Build history of the part. All positions in model axes, mm. Coordinates: 2 decimals unless noted, no trailing zeros. Loops run counter-clockwise (first coordinate to the right, second up) from the corner with the lowest first, then second, coordinate; pieces in that order, holes last.
Item 1: Cut at B-B (y = 0.5). Count the separate pieces of the cut face and the enclosed holes in it, and give its area (3 significant figures).
Item 2: Drill centre lines: line 1 along X through (y, z) = (0.7, -80.5); line 2 along Z through (x, y) = (-36.5, 2.55); line 3 along Z through (x, y) = (-81, 2.4). Where is each one in solid material? Low to high.
Item 3: Cut at A-A (z = -94.5). List the corners of the cut face in (x, y), and give its area (3 significant figures).
Item 4: Mould opens along Z. For faces 1 (the face through (-70.09, 1.48, 41.65)), 2 (the face through (2, 0, 24)), 3 (the face through (-17.75, 1.479, -38.065)) say: released by +Z, released by -Z, zero draft, split by the parting line, or undercut.
Item 5: Flat gauge pin, fed straight in: pin 1 (1.5 mm diameter, centred on x = 5, y = 2.5, fed in from +Z). Where does the tip first touch, or does it go through?
from build123d import *

# Parameters (mm, degrees)
SKETCH1_R           = 115
SKETCH1_R_2         = 1.5
SKETCH1_R_3         = 2
SKETCH1_R_4         = 15
BOSS_EXTRUDE3_DEPTH = 3


with BuildPart() as part:
    # Sketch1 → Boss-Extrude3 (new body)
    with BuildSketch(Plane(origin=(0, 0, 0), x_dir=(1, 0, 0), z_dir=(0, 1, 0))):
        with Locations(Location((0, 0, 0), (0, 0, 270))):
            Circle(SKETCH1_R)
        with Locations(Location((-65, 65, 0), (0, 0, 270))):
            Circle(SKETCH1_R_2, mode=Mode.SUBTRACT)
        with Locations(Location((-47.039487758, 27.039487758, 0), (0, 0, 270))):
            Circle(SKETCH1_R_2, mode=Mode.SUBTRACT)
        with Locations(Location((65, 65, 0), (0, 0, 270))):
            Circle(SKETCH1_R_2, mode=Mode.SUBTRACT)
        with Locations(Location((27.039487758, 47.039487758, 0), (0, 0, 270))):
            Circle(SKETCH1_R_2, mode=Mode.SUBTRACT)
        with Locations(Location((15.25, 15.25, 0), (0, 0, 270))):
            Circle(SKETCH1_R_2, mode=Mode.SUBTRACT)
        with Locations(Location((22, 22, 0), (0, 0, 270))):
            Circle(SKETCH1_R_3, mode=Mode.SUBTRACT)
        with Locations(Location((37.039487758, 55.539487758, 0), (0, 0, 270))):
            Circle(SKETCH1_R_2, mode=Mode.SUBTRACT)
        with Locations(Location((37.039487758, 38.539487758, 0), (0, 0, 270))):
            Circle(SKETCH1_R_2, mode=Mode.SUBTRACT)
        with Locations(Location((65, -65, 0), (0, 0, 270))):
            Circle(SKETCH1_R_2, mode=Mode.SUBTRACT)
        with Locations(Location((47.039487758, -27.039487758, 0), (0, 0, 270))):
            Circle(SKETCH1_R_2, mode=Mode.SUBTRACT)
        with Locations(Location((15.25, -15.25, 0), (0, 0, 270))):
            Circle(SKETCH1_R_2, mode=Mode.SUBTRACT)
        with Locations(Location((22, -22, 0), (0, 0, 270))):
            Circle(SKETCH1_R_3, mode=Mode.SUBTRACT)
        with Locations(Location((55.539487758, -37.039487758, 0), (0, 0, 270))):
            Circle(SKETCH1_R_2, mode=Mode.SUBTRACT)
        with Locations(Location((38.539487758, -37.039487758, 0), (0, 0, 270))):
            Circle(SKETCH1_R_2, mode=Mode.SUBTRACT)
        with Locations(Location((-65, -65, 0), (0, 0, 270))):
            Circle(SKETCH1_R_2, mode=Mode.SUBTRACT)
        with Locations(Location((0, 0, 0), (0, 0, 270))):
            Circle(SKETCH1_R_4, mode=Mode.SUBTRACT)
        with Locations(Location((-15.25, 15.25, 0), (0, 0, 270))):
            Circle(SKETCH1_R_2, mode=Mode.SUBTRACT)
        with Locations(Location((-22, 22, 0), (0, 0, 270))):
            Circle(SKETCH1_R_3, mode=Mode.SUBTRACT)
        with Locations(Location((-55.539487758, 37.039487758, 0), (0, 0, 270))):
            Circle(SKETCH1_R_2, mode=Mode.SUBTRACT)
        with Locations(Location((-27.039487758, -47.039487758, 0), (0, 0, 270))):
            Circle(SKETCH1_R_2, mode=Mode.SUBTRACT)
        with Locations(Location((-15.25, -15.25, 0), (0, 0, 270))):
            Circle(SKETCH1_R_2, mode=Mode.SUBTRACT)
        with Locations(Location((-22, -22, 0), (0, 0, 270))):
            Circle(SKETCH1_R_3, mode=Mode.SUBTRACT)
        with Locations(Location((-37.039487758, -55.539487758, 0), (0, 0, 270))):
            Circle(SKETCH1_R_2, mode=Mode.SUBTRACT)
        with Locations(Location((-37.039487758, -38.539487758, 0), (0, 0, 270))):
            Circle(SKETCH1_R_2, mode=Mode.SUBTRACT)
        with Locations(Location((29, 24.5, 0), (0, 0, 90))):
            Circle(SKETCH1_R_2, mode=Mode.SUBTRACT)
        with Locations(Location((29, -24.5, 0), (0, 0, 270))):
            Circle(SKETCH1_R_2, mode=Mode.SUBTRACT)
        with Locations(Location((-29, -24.5, 0), (0, 0, 90))):
            Circle(SKETCH1_R_2, mode=Mode.SUBTRACT)
        with Locations(Location((-29, 24.5, 0), (0, 0, 270))):
            Circle(SKETCH1_R_2, mode=Mode.SUBTRACT)
        with Locations(Location((-38.539487758, 37.039487758, 0), (0, 0, 270))):
            Circle(SKETCH1_R_2, mode=Mode.SUBTRACT)
        with BuildLine():
            Line((26.808945881, 12.501216771), (49.6405219, 23.147755517))
            ThreePointArc((49.6405219, 23.147755517), (53.675730643, 23.232000867), (56.458487137, 20.308599907))
            ThreePointArc((56.458487137, 20.308599907), (60, 0), (56.458487137, -20.308599907))
            ThreePointArc((56.458487137, -20.308599907), (53.675730643, -23.232000867), (49.6405219, -23.147755517))
            Line((49.6405219, -23.147755517), (26.808945881, -12.501216771))
            ThreePointArc((26.808945881, -12.501216771), (24.383041239, -10.066703292), (24.101697658, -6.641398197))
            ThreePointArc((24.101697658, -6.641398197), (25, 0), (24.101697658, 6.641398197))
            ThreePointArc((24.101697658, 6.641398197), (24.383041239, 10.066703292), (26.808945881, 12.501216771))
        make_face(mode=Mode.SUBTRACT)
        with BuildLine():
            Line((67.821864521, 31.625854817), (90.517419336, 42.208965833))
            ThreePointArc((90.517419336, 42.208965833), (94.457574862, 42.331654691), (97.262036177, 39.561298243))
            ThreePointArc((97.262036177, 39.561298243), (104.05397345, -14.063093872), (83.270844776, -63.960662992))
            ThreePointArc((83.270844776, -63.960662992), (78.486399596, -65.847357267), (74.568650349, -62.515425125))
            Line((74.568650349, -62.515425125), (64.070056019, -31.443439938))
            ThreePointArc((64.070056019, -31.443439938), (63.811318327, -29.63450173), (64.219840648, -27.853403152))
            ThreePointArc((64.219840648, -27.853403152), (69.986267395, -1.386497808), (65.272625441, 25.288028156))
            ThreePointArc((65.272625441, 25.288028156), (65.296141705, 28.960167834), (67.821864521, 31.625854817))
        make_face(mode=Mode.SUBTRACT)
        with BuildLine():
            Line((12.501216771, -26.808945881), (23.147755517, -49.6405219))
            ThreePointArc((23.147755517, -49.6405219), (23.232000867, -53.675730643), (20.308599907, -56.458487137))
            ThreePointArc((20.308599907, -56.458487137), (0, -60), (-20.308599907, -56.458487137))
            ThreePointArc((-20.308599907, -56.458487137), (-23.232000867, -53.675730643), (-23.147755517, -49.6405219))
            Line((-23.147755517, -49.6405219), (-12.501216771, -26.808945881))
            ThreePointArc((-12.501216771, -26.808945881), (-10.066703292, -24.383041239), (-6.641398197, -24.101697658))
            ThreePointArc((-6.641398197, -24.101697658), (0, -25), (6.641398197, -24.101697658))
            ThreePointArc((6.641398197, -24.101697658), (10.066703292, -24.383041239), (12.501216771, -26.808945881))
        make_face(mode=Mode.SUBTRACT)
        with BuildLine():
            Line((-26.808945881, -12.501216771), (-49.6405219, -23.147755517))
            ThreePointArc((-49.6405219, -23.147755517), (-53.675730643, -23.232000867), (-56.458487137, -20.308599907))
            ThreePointArc((-56.458487137, -20.308599907), (-60, 0), (-56.458487137, 20.308599907))
            ThreePointArc((-56.458487137, 20.308599907), (-53.675730643, 23.232000867), (-49.6405219, 23.147755517))
            Line((-49.6405219, 23.147755517), (-26.808945881, 12.501216771))
            ThreePointArc((-26.808945881, 12.501216771), (-24.383041239, 10.066703292), (-24.101697658, 6.641398197))
            ThreePointArc((-24.101697658, 6.641398197), (-25, 0), (-24.101697658, -6.641398197))
            ThreePointArc((-24.101697658, -6.641398197), (-24.383041239, -10.066703292), (-26.808945881, -12.501216771))
        make_face(mode=Mode.SUBTRACT)
        with BuildLine():
            Line((-12.501216771, 26.808945881), (-23.147755517, 49.6405219))
            ThreePointArc((-23.147755517, 49.6405219), (-23.232000867, 53.675730643), (-20.308599907, 56.458487137))
            ThreePointArc((-20.308599907, 56.458487137), (0, 60), (20.308599907, 56.458487137))
            ThreePointArc((20.308599907, 56.458487137), (23.232000867, 53.675730643), (23.147755517, 49.6405219))
            Line((23.147755517, 49.6405219), (12.501216771, 26.808945881))
            ThreePointArc((12.501216771, 26.808945881), (10.066703292, 24.383041239), (6.641398197, 24.101697658))
            ThreePointArc((6.641398197, 24.101697658), (0, 25), (-6.641398197, 24.101697658))
            ThreePointArc((-6.641398197, 24.101697658), (-10.066703292, 24.383041239), (-12.501216771, 26.808945881))
        make_face(mode=Mode.SUBTRACT)
        with BuildLine():
            Line((31.625854817, -67.821864521), (42.208965833, -90.517419336))
            ThreePointArc((42.208965833, -90.517419336), (42.331654691, -94.457574862), (39.561298243, -97.262036177))
            ThreePointArc((39.561298243, -97.262036177), (-14.063093872, -104.05397345), (-63.960662992, -83.270844776))
            ThreePointArc((-63.960662992, -83.270844776), (-65.847357267, -78.486399596), (-62.515425125, -74.568650349))
            Line((-62.515425125, -74.568650349), (-31.443439938, -64.070056019))
            ThreePointArc((-31.443439938, -64.070056019), (-29.63450173, -63.811318327), (-27.853403152, -64.219840648))
            ThreePointArc((-27.853403152, -64.219840648), (-1.386497808, -69.986267395), (25.288028156, -65.272625441))
            ThreePointArc((25.288028156, -65.272625441), (28.960167834, -65.296141705), (31.625854817, -67.821864521))
        make_face(mode=Mode.SUBTRACT)
        with BuildLine():
            Line((-67.821864521, -31.625854817), (-90.517419336, -42.208965833))
            ThreePointArc((-90.517419336, -42.208965833), (-94.457574862, -42.331654691), (-97.262036177, -39.561298243))
            ThreePointArc((-97.262036177, -39.561298243), (-104.05397345, 14.063093872), (-83.270844776, 63.960662991))
            ThreePointArc((-83.270844776, 63.960662991), (-78.486399596, 65.847357267), (-74.568650349, 62.515425125))
            Line((-74.568650349, 62.515425125), (-64.070056019, 31.443439938))
            ThreePointArc((-64.070056019, 31.443439938), (-63.811318327, 29.63450173), (-64.219840648, 27.853403152))
            ThreePointArc((-64.219840648, 27.853403152), (-69.986267395, 1.386497808), (-65.272625441, -25.288028156))
            ThreePointArc((-65.272625441, -25.288028156), (-65.296141705, -28.960167834), (-67.821864521, -31.625854817))
        make_face(mode=Mode.SUBTRACT)
        with BuildLine():
            Line((-31.625854817, 67.821864521), (-42.208965833, 90.517419336))
            ThreePointArc((-42.208965833, 90.517419336), (-42.331654691, 94.457574862), (-39.561298243, 97.262036177))
            ThreePointArc((-39.561298243, 97.262036177), (14.063093872, 104.05397345), (63.960662992, 83.270844776))
            ThreePointArc((63.960662992, 83.270844776), (65.847357267, 78.486399596), (62.515425125, 74.568650349))
            Line((62.515425125, 74.568650349), (31.443439938, 64.070056019))
            ThreePointArc((31.443439938, 64.070056019), (29.63450173, 63.811318327), (27.853403152, 64.219840648))
            ThreePointArc((27.853403152, 64.219840648), (1.386497808, 69.986267395), (-25.288028156, 65.272625441))
            ThreePointArc((-25.288028156, 65.272625441), (-28.960167834, 65.296141705), (-31.625854817, 67.821864521))
        make_face(mode=Mode.SUBTRACT)
        with BuildLine():
            ThreePointArc((-45.978827586, 45.978827586), (-38.640025446, 70.362997436), (-54.923082637, 89.941245688))
            ThreePointArc((-54.923082637, 89.941245688), (-56.875768309, 89.112379796), (-56.046902417, 87.159694124))
            ThreePointArc((-56.046902417, 87.159694124), (-41.57979956, 69.764893633), (-48.10014793, 48.10014793))
            ThreePointArc((-48.10014793, 48.10014793), (-48.10014793, 45.978827586), (-45.978827586, 45.978827586))
        make_face(mode=Mode.SUBTRACT)
        with BuildLine():
            ThreePointArc((45.978827586, 45.978827586), (70.362997436, 38.640025446), (89.941245688, 54.923082637))
            ThreePointArc((89.941245688, 54.923082637), (89.112379796, 56.875768309), (87.159694124, 56.046902417))
            ThreePointArc((87.159694124, 56.046902417), (69.764893633, 41.57979956), (48.10014793, 48.10014793))
            ThreePointArc((48.10014793, 48.10014793), (45.978827586, 48.10014793), (45.978827586, 45.978827586))
        make_face(mode=Mode.SUBTRACT)
        with BuildLine():
            ThreePointArc((45.978827586, -45.978827586), (38.640025446, -70.362997436), (54.923082637, -89.941245688))
            ThreePointArc((54.923082637, -89.941245688), (56.875768309, -89.112379796), (56.046902417, -87.159694124))
            ThreePointArc((56.046902417, -87.159694124), (41.57979956, -69.764893633), (48.10014793, -48.10014793))
            ThreePointArc((48.10014793, -48.10014793), (48.10014793, -45.978827586), (45.978827586, -45.978827586))
        make_face(mode=Mode.SUBTRACT)
        with BuildLine():
            ThreePointArc((-45.978827586, -45.978827586), (-70.362997436, -38.640025446), (-89.941245688, -54.923082637))
            ThreePointArc((-89.941245688, -54.923082637), (-89.112379796, -56.875768309), (-87.159694124, -56.046902417))
            ThreePointArc((-87.159694124, -56.046902417), (-69.764893633, -41.57979956), (-48.10014793, -48.10014793))
            ThreePointArc((-48.10014793, -48.10014793), (-45.978827586, -48.10014793), (-45.978827586, -45.978827586))
        make_face(mode=Mode.SUBTRACT)
    extrude(amount=BOSS_EXTRUDE3_DEPTH)


solid = part.part
Filled sheet:
1. separate pieces: 1
1. enclosed holes: 41
1. area: 22,000 mm2
2. line 1: x = -82.13 to -46.81, -43.01 to -37.54, 65.77 to 82.13
2. line 2: z = -109.05 to -98.45, -78.27 to -17.02, 17.02 to 37.14, 39.94 to 54.14, 56.94 to 65.78, 98.45 to 109.05
2. line 3: z = -81.63 to -65.62, 37.77 to 43.38, 47.25 to 81.63
3. outline: (-65.53, 0) - (-42.31, 0) - (-42.31, 3) - (-65.53, 3) - close; (45.77, 0) - (65.53, 0) - (65.53, 3) - (45.77, 3) - close
3. area: 129 mm2
4. face 1: undercut
4. face 2: zero draft
4. face 3: undercut
5. pin 1: stops at z = 114.92
